For this review, use the dimensioned drawing (mm, ordinates from the lowest corner) and the shaded views. Coordinates: 2 decimals unless noted, no trailing zeros. Loops run counter-clockwise (first coordinate to the right, second up) from the corner with the lowest first, then second, coordinate; pieces in that order, holes last.
1. Take a section at D-D, the plane x = 48.5. State the section outline as (y, z) points, then the cut area to 3 significant figures.
2. Take a section at B-B, the plane z = 40. State the section outline as (x, y) points.
3. Take a section at C-C, the plane y = 1.55. State the section outline as (x, z) points.
4. Clearance check with a flat-ended pin moving along its axis: P1, Ø3, axis at x = 114.5, z = 58.5, coming from the -Y side. State where the tip first meets the part, or that it passes through.
5. Take a section at A-A, the plane x = 30. State the section outline as (y, z) points, then the cut area to 3 significant figures.
6. To check wall thickness, follow probe 1 along X at (y, z) = (1.6, 40); probe 2 along Z at (x, y) = (48.5, 0.95); probe 3 along Z at (x, y) = (30, 0.45). State the ranges of each line that lie inside material, in increasing order.
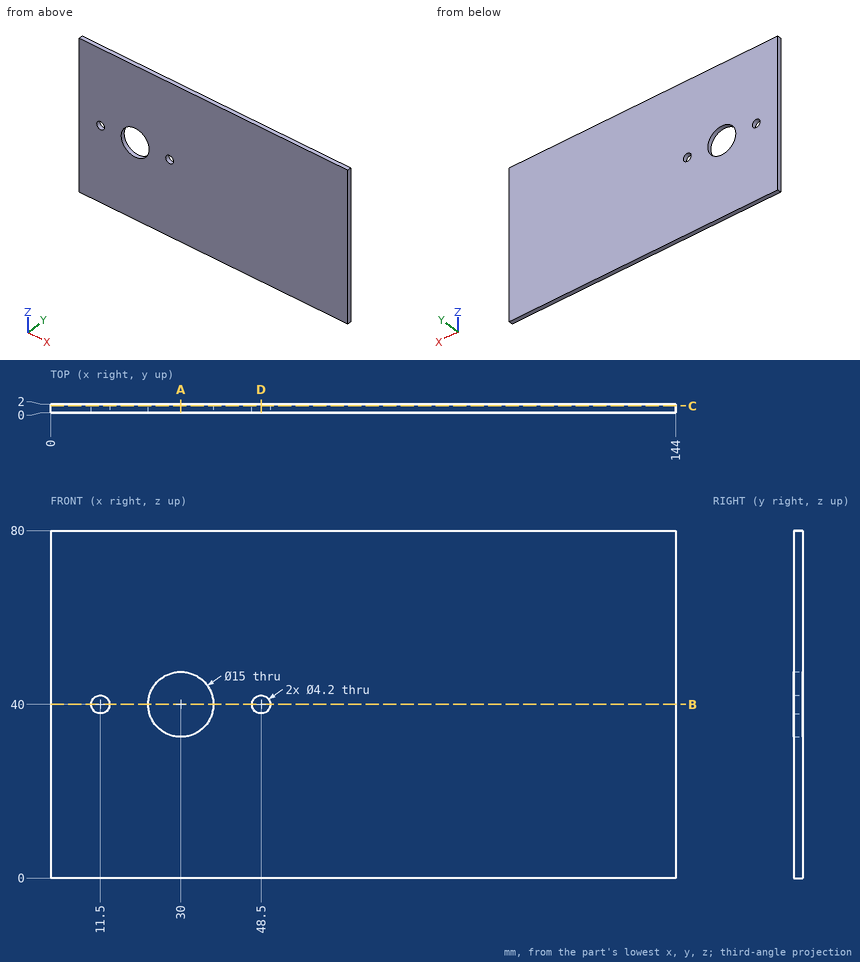
Results list:
1. outline: (0, 0) - (2, 0) - (2, 37.9) - (0, 37.9) - close; (0, 42.1) - (2, 42.1) - (2, 80) - (0, 80) - close
1. area: 152 mm2
2. outline: (0, 0) - (9.4, 0) - (9.4, 2) - (0, 2) - close; (13.6, 0) - (22.5, 0) - (22.5, 2) - (13.6, 2) - close; (37.5, 0) - (46.4, 0) - (46.4, 2) - (37.5, 2) - close; (50.6, 0) - (144, 0) - (144, 2) - (50.6, 2) - close
3. outline: (0, 0) - (144, 0) - (144, 80) - (0, 80) - close; hole circle Ø4.2 at (11.5, 40); hole circle Ø15 at (30, 40); hole circle Ø4.2 at (48.5, 40)
4. P1: stops at y = 0
5. outline: (0, 0) - (2, 0) - (2, 32.5) - (0, 32.5) - close; (0, 47.5) - (2, 47.5) - (2, 80) - (0, 80) - close
5. area: 130 mm2
6. probe 1: x = 0 to 9.4, 13.6 to 22.5, 37.5 to 46.4, 50.6 to 144
6. probe 2: z = 0 to 37.9, 42.1 to 80
6. probe 3: z = 0 to 32.5, 47.5 to 80
